Study the drawing (mm; zero at the part's minimum x, y, z) and answer. A direction names the side the tool comes from. Give positions to 0.01 mm unless a question says otherwise; leave off trailing zeros. Write each loop counter-clockwise with the first axis right and the second up, starting at its lowest first coordinate (ties: lowest second). Pieces come first, ordered by that corner, then holes. Notation, with made-up numbers: (45, 30) -> (84, 30) arc R14 ccw to (84, 48) -> close; hole circle Ø5 at (42, 79.25). An arc over 180 degrees is marked (long way). One line per question, with ' | ' between items.
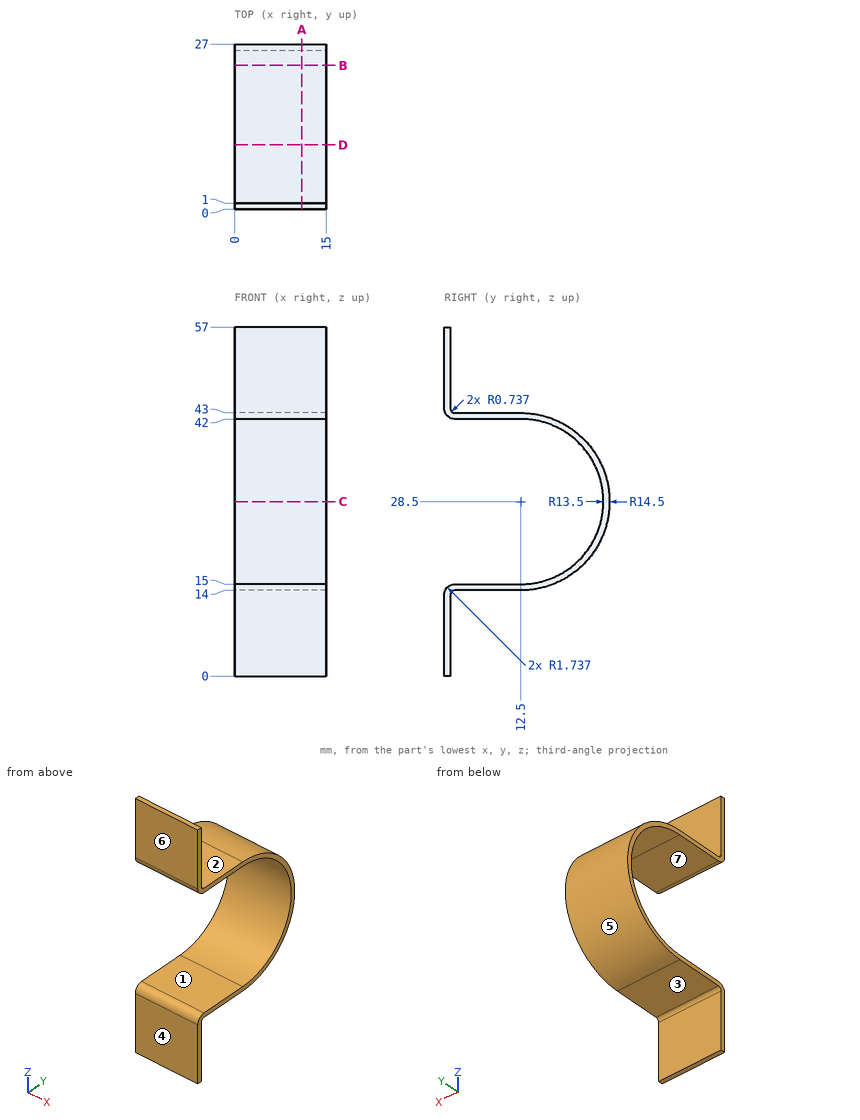
Item 1: Determine the mould class of the marked faces 5, 6 and 7 for opening direction Z: pulls with the +Z half, pulls with the -Z half, needs draft (parallel to the pull), parting line crosses it, or undercut.
Answers below:
face 5: parting line crosses it | face 6: needs draft | face 7: undercut
Item 2: A tool of negligible diameter and unlimited length cuts with its end or side. For the marked faces 1, 2, 3 and 4, from which of +Z, -Z, +X, -X, +Y, -Y can it reach the whole face along a straight path? Write none if from no direction.
Answers below:
face 1: +X, -X, -Y | face 2: +Z, +X, -X, +Y | face 3: -Z, +X, -X, +Y | face 4: +Z, -Z, +X, -X, -Y
Item 3: Flat-ended cylindrical pins translate along their axes: pin 1 (4 mm diameter, centred on x = 7.5, z = 6.5, fed in from +Y); pin 2 (3 mm diameter, centred on x = 10.5, y = 7, fed in from -Z); pin 3 (5 mm diameter, centred on x = 3, z = 27, fed in from -Y). Find the tip coordinate at first contact, or state that the pin passes through.
Answers below:
pin 1: y = 1 | pin 2: z = 14 | pin 3: y = 25.39
Item 4: Find section D-D (y = 10.5). Write down the section's boundary in (x, z).
Answers below:
outline: (0, 14) -> (15, 14) -> (15, 15) -> (0, 15) -> close; (0, 42) -> (15, 42) -> (15, 43) -> (0, 43) -> close
Item 5: Find section B-B (y = 23.5). Write down the section's boundary in (x, z).
Answers below:
outline: (0, 19.05) -> (15, 19.05) -> (15, 20.67) -> (0, 20.67) -> close; (0, 36.33) -> (15, 36.33) -> (15, 37.95) -> (0, 37.95) -> close
Item 6: Find section C-C (z = 28.5). Write down the section's boundary in (x, y), then the cut area to 3 significant figures.
Answers below:
outline: (0, 26) -> (15, 26) -> (15, 27) -> (0, 27) -> close | area: 15.0 mm²
Item 7: Consider line 1 (Z direction, x = 0.5, y = 7.75); line 2 (Z direction, x = 11, y = 14.5); line 3 (Y direction, x = 4, z = 13). Determine where each line is inside the solid, lowest interval first. Write a range as [from, to].
Answers below:
line 1: [14, 15], [42, 43] | line 2: [14.14, 15.15], [41.85, 42.86] | line 3: [0, 1]
Item 8: Find section A-A (x = 11). Write down the section's boundary in (y, z).
Answers below:
outline: (0, 0) -> (1, 0) -> (1, 13.26) arc R0.74 cw to (1.74, 14) -> (12.5, 14) arc R14.5 ccw to (12.5, 43) -> (1.74, 43) arc R0.74 cw to (1, 43.74) -> (1, 57) -> (0, 57) -> (0, 43.74) arc R1.74 ccw to (1.74, 42) -> (12.5, 42) arc R13.5 cw to (12.5, 15) -> (1.74, 15) arc R1.74 ccw to (0, 13.26) -> close
